Here's the drawing with two shaded views (mm, measured from the low corner). I have some questions. A direction names the side the tool comes from. Round coordinates to 2 decimals unless told otherwise and drop trailing zeros. Loops run counter-clockwise (first coordinate to the right, second up) from the corner with the lowest first, then second, coordinate; pieces in that order, holes last.
(1) If I drill on line 1 along Z through (x, y) = (3.35, 1.7); line 2 along Y through (x, z) = (2.5, 7.25); line 3 along Z through (x, y) = (2, 0.2), over which ranges is the centre line in solid material (lowest first)?
(2) I want a section at A-A on x = 3.35. Write out the boundary of the cut face in (y, z).
(3) I want a section at D-D on y = 1. Write out the boundary of the cut face in (x, z).
(4) I want a section at C-C on y = 1.9. Write out the boundary of the cut face in (x, z).
(5) Will this pin go through, and if not, where does the flat tip stop? pin 1 Ø0.8 at (x, y) = (4, 1) entering from -Z.
(6) I want a section at B-B on x = 6.25. Write out the boundary of the cut face in (y, z).
(7) Which directions (+Z, -Z, +X, -X, +Y, -Y) give clear straight access to the entire face, cutting with the end or side of a thin tool? Please do the marked faces 1 and 2.
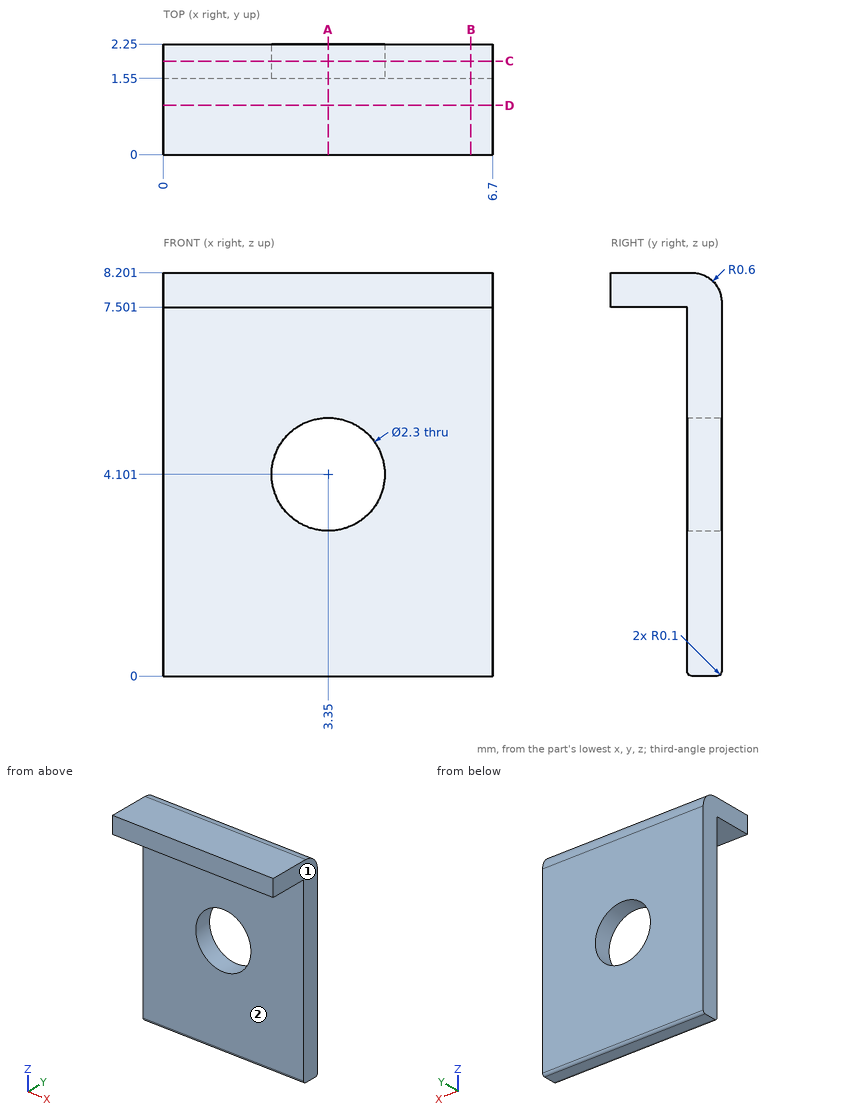
Filled sheet:
1. line 1: z = 0 to 2.95, 5.25 to 8.2
1. line 2: y = 1.55 to 2.25
1. line 3: z = 7.5 to 8.2
2. outline: (0, 7.5) - (1.55, 7.5) - (1.55, 5.25) - (2.25, 5.25) - (2.25, 7.6) arc R0.6 ccw to (1.65, 8.2) - (0, 8.2) - close; (1.55, 0.1) arc R0.1 ccw to (1.65, 0) - (2.15, 0) arc R0.1 ccw to (2.25, 0.1) - (2.25, 2.95) - (1.55, 2.95) - close
3. outline: (0, 7.5) - (6.7, 7.5) - (6.7, 8.2) - (0, 8.2) - close
4. outline: (0, 0) - (6.7, 0) - (6.7, 8.15) - (0, 8.15) - close; hole circle Ø2.3 at (3.35, 4.1)
5. pin 1: stops at z = 7.5
6. outline: (0, 7.5) - (1.55, 7.5) - (1.55, 0.1) arc R0.1 ccw to (1.65, 0) - (2.15, 0) arc R0.1 ccw to (2.25, 0.1) - (2.25, 7.6) arc R0.6 ccw to (1.65, 8.2) - (0, 8.2) - close
7. face 1: +Z, -Z, +X, +Y, -Y
7. face 2: -Z, +X, -X, -Y
